Build history of the part. All positions in model axes, mm. Round coordinates to 2 decimals unless told otherwise and drop trailing zeros. Write each loop counter-clockwise with the first axis right and the second up, starting at its lowest first coordinate (ties: lowest second). Pieces come first, ordered by that corner, then holes. Notation, with made-up numbers: (26.5, -22) - (61.5, -22) arc R26 ccw to (61.5, 15) - close; hole circle Ø11 at (63, 59). An arc over 180 degrees is marked (long way). Answer as a JSON object with one key per item and string values. Group by question number.
Item 1: Flat gauge pins, fed straight in: pin 1 (8 mm diameter, centred on x = 331, z = -4, fed in from -Y); pin 2 (12 mm diameter, centred on x = 240, z = 0.5, fed in from +Y); pin 3 (15 mm diameter, centred on x = 457.2, z = 0, fed in from -Y); pin 4 (2 mm diameter, centred on x = 344.5, z = 5, fed in from +Y). Where does each tip first touch, or does it go through?
Item 2: Probe line 1 (Z direction, x = -457.2, y = -18.5); line 2 (X direction, y = 13, z = -25); line 3 (X direction, y = -6, z = -39). List the from-to ranges inside material, lowest first. Write a range as from..to.
Item 3: Slice it at A-A, the plane x = 110.5. List the corners of the cut face in (y, z) (1 decimal).
from build123d import *

# Parameters (mm, degrees)
F0_W     = 431.8
F0_H     = 12.7
F0_H_2   = 4.7625
F3_DEPTH = 25.4


with BuildPart() as f1:
    # F0 (on Front) → F1 (revolve)
    with BuildSketch(Plane.XZ):
        with Locations((-215.9, 6.35)):
            Rectangle(F0_W, F0_H)
    revolve(axis=Axis((-228.6, 0, 0), (1, 0, 0)))



with BuildPart() as f2:
    # F0 (on Front) → F2 (revolve)
    with BuildSketch(Plane.XZ):
        with Locations((-215.9, -23.01875)):
            Rectangle(F0_W, F0_H_2)
    revolve(axis=Axis((-228.6, 0, -25.4), (-1, 0, 0)))


with BuildPart() as f1_1:
    add(f1.part)

    add(f2.part)  # F3 merges F2
    # F0 (on Front) → F3 (join, symmetric)
    with BuildSketch(Plane.XZ):
        with BuildLine():
            Line((-431.8, 0), (-444.5, 0))
            ThreePointArc((-444.5, 0), (-466.1802561211, -8.9802561211), (-457.2, 12.7))
            Line((-457.2, 12.7), (-431.8, 12.7))
            Line((-431.8, 12.7), (-431.8, 25.4))
            Line((-431.8, 25.4), (-482.6, 25.4))
            Line((-482.6, 25.4), (-482.6, -44.45))
            Line((-482.6, -44.45), (-431.8, -44.45))
            Line((-431.8, -44.45), (-431.8, -25.4))
            Line((-431.8, -25.4), (-452.4375, -25.4))
            ThreePointArc((-452.4375, -25.4), (-460.5675960454, -28.7675960454), (-457.2, -20.6375))
            Line((-457.2, -20.6375), (-431.8, -20.6375))
            Line((-431.8, -20.6375), (-431.8, 0))
        make_face()
        with BuildLine():
            ThreePointArc((-457.2, 12.7), (-448.2197438789, 8.9802561211), (-444.5, 0))
            Line((-444.5, 0), (-431.8, 0))
            Line((-431.8, 0), (-431.8, 12.7))
            Line((-431.8, 12.7), (-457.2, 12.7))
        make_face()
        with BuildLine():
            Line((-431.8, -25.4), (-431.8, -20.6375))
            Line((-431.8, -20.6375), (-457.2, -20.6375))
            ThreePointArc((-457.2, -20.6375), (-453.8324039546, -22.0324039546), (-452.4375, -25.4))
            Line((-452.4375, -25.4), (-431.8, -25.4))
        make_face()
    extrude(amount=F3_DEPTH, both=True)

    # F4: F1 across plane


with BuildPart() as f1_2:
    add(f1_1.part)
    add(f1_1.part.mirror(Plane.YZ))


solid = f1_2.part
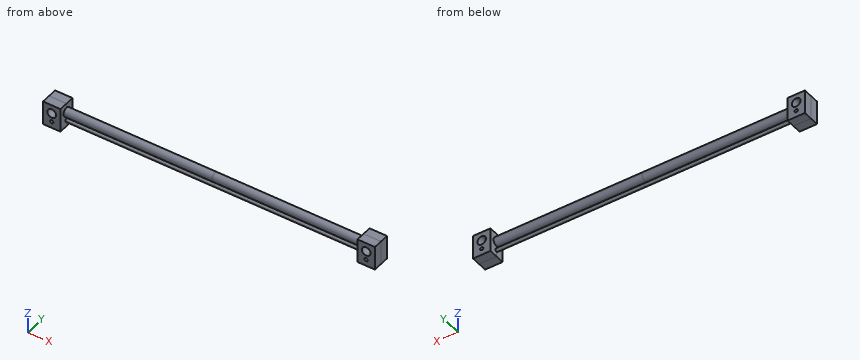
Geometry says:
{
 "1": {"pin 1": "stops at y = -12.7", "pin 2": "stops at y = 12.7", "pin 3": "passes through", "pin 4": "stops at y = 12.05"},
 "2": {"line 1": "z = -44.45..-30.16, -20.64..-12.7, 12.7..25.4", "line 2": "x = -482.6..-461.95, -452.45..-431.8, 431.8..452.45, 461.95..482.6", "line 3": "x = -482.6..-431.8, 431.8..482.6"},
 "3": {"outline": "circle Ø25.4 at (0, 0); circle Ø9.5 at (0, -25.4)"}
}
